Source: CAD feature listing. Evaluate the final solid. Frame: model axes, mm. A direction names the side the tool comes from. Give positions to 0.01 mm unless a question says otherwise; leave off trailing zeros. Loops run counter-clockwise (first coordinate to the right, second up) from the corner with the lowest first, then second, coordinate; pieces in that order, holes last. Notation, with made-up numbers: M 75.5,9.5 L 128.5,9.5 A17 ccw 128.5,27.5 Z; hole C 59.25,75.5 d7. An arc over 180 degrees is marked long. Answer in a Markdown table with one row per item.
```python
from build123d import *

# Parameters (mm, degrees)
BOSS_EXTRUDE1_DEPTH = 20
SKETCH2_R           = 1.35
CUT_EXTRUDE2_DEPTH  = 12
SKETCH3_R           = 10
BOSS_EXTRUDE2_DEPTH = 6
SKETCH4_R           = 1.35
CUT_EXTRUDE3_DEPTH  = 10


with BuildPart() as part:
    # Sketch1 → Boss-Extrude1 (new body)
    with BuildSketch(Plane.XY):
        with BuildLine():
            Line((-5, -19.5), (3, -19.5))
            ThreePointArc((3, -19.5), (4.414213562, -18.914213562), (5, -17.5))
            Line((5, -17.5), (5, 17.5))
            ThreePointArc((5, 17.5), (4.414213562, 18.914213562), (3, 19.5))
            Line((3, 19.5), (-5, 19.5))
            Line((-5, 19.5), (-5, -19.5))
        make_face()
    extrude(amount=BOSS_EXTRUDE1_DEPTH)

    # Sketch2 → Cut-Extrude2 (cut)
    with BuildSketch(Plane.XY.offset(20)):
        with Locations((-0.5, 15.5)):
            Circle(SKETCH2_R)
        with Locations((-0.5, 5.5)):
            Circle(SKETCH2_R)
        with Locations((-0.5, -15.5)):
            Circle(SKETCH2_R)
        with Locations((-0.5, -5.5)):
            Circle(SKETCH2_R)
    extrude(amount=-CUT_EXTRUDE2_DEPTH, mode=Mode.SUBTRACT)

    # Sketch3 → Boss-Extrude2 (add)
    with BuildSketch(Plane(origin=(5, 0, 0), x_dir=(0, 0, -1), z_dir=(1, 0, 0))):
        with Locations((-10, 0)):
            Circle(SKETCH3_R)
    extrude(amount=BOSS_EXTRUDE2_DEPTH)

    # Sketch4 → Cut-Extrude3 (cut)
    with BuildSketch(Plane(origin=(11, 0, 0), x_dir=(0, 0, -1), z_dir=(1, 0, 0))):
        with Locations((-17, 0)):
            Circle(SKETCH4_R)
        with Locations((-10, 7)):
            Circle(SKETCH4_R)
        with Locations((-3, 0)):
            Circle(SKETCH4_R)
        with Locations((-10, -7)):
            Circle(SKETCH4_R)
    extrude(amount=-CUT_EXTRUDE3_DEPTH, mode=Mode.SUBTRACT)


solid = part.part
```
1) Section C-C, the plane x = -0.5. Return loops of the section in (y, z).
Reply:
| item | result |
|---|---|
| outline | M -19.5,0 L 19.5,0 L 19.5,20 L 16.85,20 L 16.85,8 L 14.15,8 L 14.15,20 L 6.85,20 L 6.85,8 L 4.15,8 L 4.15,20 L -4.15,20 L -4.15,8 L -6.85,8 L -6.85,20 L -14.15,20 L -14.15,8 L -16.85,8 L -16.85,20 L -19.5,20 Z |
2) Section A-A, the plane z = 10. Return loops of the section in (x, y), then the cut area to 3 significant figures.
Reply:
| item | result |
|---|---|
| outline | M -5,-19.5 L 3,-19.5 A2 ccw 5,-17.5 L 5,-10 L 11,-10 L 11,-8.35 L 1,-8.35 L 1,-5.65 L 11,-5.65 L 11,5.65 L 1,5.65 L 1,8.35 L 11,8.35 L 11,10 L 5,10 L 5,17.5 A2 ccw 3,19.5 L -5,19.5 Z; hole C -0.5,-15.5 d2.7; hole C -0.5,-5.5 d2.7; hole C -0.5,5.5 d2.7; hole C -0.5,15.5 d2.7 |
| area | 431 mm² |
3) Pin query (flat end, axial travel): pin 1 Ø1.5 at (x, z) = (8, 3) entering from +Y; pin 2 Ø2 at (x, y) = (8, -6.5) entering from +Z; pin 3 Ø1.6 at (y, z) = (0, 17) entering from +X. Return the tip coordinate at first contact, or that it passes through.
Reply:
| item | result |
|---|---|
| pin 1 | stops at y = 7.81 |
| pin 2 | stops at z = 18.35 |
| pin 3 | stops at x = 1 |
4) Material intervals for L1, parallel to Y at x = -0.5, z = 13.5; L2, parallel to Y at x = 6.75, z = 10; L3, parallel to Y at x = 1.75, z = 3, sorted ascending.
Reply:
| item | result |
|---|---|
| L1 | y = -19.5 to -16.85, -14.15 to -6.85, -4.15 to 4.15, 6.85 to 14.15, 16.85 to 19.5 |
| L2 | y = -10 to -8.35, -5.65 to 5.65, 8.35 to 10 |
| L3 | y = -19.5 to -1.35, 1.35 to 19.5 |
5) Set-up query: faces 1 (the cylindrical face through (6.07, -5.862, 9.274)), 2 (the flat face through (0, 0, 20)), 3 (the cylindrical face through (0.226, -4.362, 14.084)). Return all of +Z, -Z, +X, -X, +Y, -Y with unobstructed straight access to the full face (end or side cutting, diameter ignored); none if empty.
Reply:
| item | result |
|---|---|
| face 1 | +X |
| face 2 | +Z, +X, -X, +Y, -Y |
| face 3 | +Z |
6) Section B-B, the plane y = -15.5. Return loops of the section in (x, z), then the cut area to 3 significant figures.
Reply:
| item | result |
|---|---|
| outline | M -5,0 L 5,0 L 5,20 L 0.85,20 L 0.85,8 L -1.85,8 L -1.85,20 L -5,20 Z |
| area | 168 mm² |
7) Section D-D, the plane z = 18.75. Return loops of the section in (x, y), then the cut area to 3 significant figures.
Reply:
| item | result |
|---|---|
| outline | M -5,-19.5 L 3,-19.5 A2 ccw 5,-17.5 L 5,-4.84 L 11,-4.84 L 11,4.84 L 5,4.84 L 5,17.5 A2 ccw 3,19.5 L -5,19.5 Z; hole C -0.5,-15.5 d2.7; hole C -0.5,-5.5 d2.7; hole C -0.5,5.5 d2.7; hole C -0.5,15.5 d2.7 |
| area | 423 mm² |
8) Pull-direction query (Y, two-part tool) for faces 4 (the flat face through (5, -13, 10)), 5 (the cylindrical face through (6.07, 8.138, 9.274)), 6 (the cylindrical face through (4.43, 18.9, 9.86)); classes: released by +Y, released by -Y, zero draft, split by the parting line, or undercut.
Reply:
| item | result |
|---|---|
| face 4 | zero draft |
| face 5 | undercut |
| face 6 | released by +Y |
